```python
from build123d import *

# Parameters (mm, degrees)
SKETCH1_W           = 88
SKETCH1_H           = 51
BOSS_EXTRUDE1_DEPTH = 2
SKETCH2_W           = 60.2
SKETCH2_H           = 45.9
CUT_EXTRUDE1_DEPTH  = 2
SKETCH3_W           = 92
SKETCH3_H           = 55
SKETCH3_W_2         = 88
SKETCH3_H_2         = 51
BOSS_EXTRUDE2_DEPTH = 26


with BuildPart() as part:
    # Sketch1 → Boss-Extrude1 (new body)
    with BuildSketch(Plane(origin=(0, 0, 0), x_dir=(1, 0, 0), z_dir=(0, 1, 0))):
        Rectangle(SKETCH1_W, SKETCH1_H)
    extrude(amount=BOSS_EXTRUDE1_DEPTH)

    # Sketch2 → Cut-Extrude1 (cut)
    with BuildSketch(Plane(origin=(0, 0, 0), x_dir=(1, 0, 0), z_dir=(0, 1, 0))):
        with Locations((-3.6, 0)):
            Rectangle(SKETCH2_W, SKETCH2_H)
    extrude(amount=CUT_EXTRUDE1_DEPTH, mode=Mode.SUBTRACT)

    # Sketch3 → Boss-Extrude2 (add)
    with BuildSketch(Plane(origin=(0, 0, 0), x_dir=(1, 0, 0), z_dir=(0, 1, 0))):
        Rectangle(SKETCH3_W, SKETCH3_H)
        Rectangle(SKETCH3_W_2, SKETCH3_H_2, mode=Mode.SUBTRACT)
    extrude(amount=BOSS_EXTRUDE2_DEPTH)


solid = part.part
```
Geometry: final body of the model. Coordinates: model frame, mm. A direction names the side the tool comes from. Round coordinates to 2 decimals unless told otherwise and drop trailing zeros. Write each loop counter-clockwise with the first axis right and the second up, starting at its lowest first coordinate (ties: lowest second). Pieces come first, ordered by that corner, then holes.
Item 1: Section query D-D (x = -38). Return loops of the section in (y, z), plus the area to 3 significant figures.
Item 2: Pin query (flat end, axial travel): P1, Ø6, axis at x = -17, z = 18, coming from the +Y side. Return the tip coordinate at first contact, or that it passes through.
Item 3: Section query B-B (x = -3). Return loops of the section in (y, z), plus the area to 3 significant figures.
Item 4: Material intervals for L1, parallel to Z at x = -4, y = 4; L2, parallel to X at y = 16.25, z = 20.5; L3, parallel to Y at x = 42, z = 7, sorted ascending.
Item 5: Mould query, pull axis X, two halves, no side actions, for faces 1 (the face through (46, 13, 0)), 2 (the face through (-4, 1, -22.95)), 3 (the face through (-46, 13, 0)), 4 (the face through (-1, 13, -27.5)). Classes: +X half, -X half, draft (parallel to the pull), parting line (faces both ways), or undercut.
Item 6: Section query C-C (z = 10.5). Return loops of the section in (x, y).
Item 7: Section query A-A (y = 23.5). Return loops of the section in (x, z).
Item 8: Set-up query: faces 5 (the face through (-4, 26, 26)), 6 (the face through (-1, 14, 25.5)), 7 (the face through (-33.7, 1, 0)). Return all of +Z, -Z, +X, -X, +Y, -Y with unobstructed straight access to the full face (end or side cutting, diameter ignored); none if empty.
Completed:
1. outline: (0, -27.5) - (26, -27.5) - (26, -25.5) - (2, -25.5) - (2, 25.5) - (26, 25.5) - (26, 27.5) - (0, 27.5) - close
1. area: 206 mm2
2. P1: passes through
3. outline: (0, -27.5) - (26, -27.5) - (26, -25.5) - (2, -25.5) - (2, -22.95) - (0, -22.95) - close; (0, 22.95) - (2, 22.95) - (2, 25.5) - (26, 25.5) - (26, 27.5) - (0, 27.5) - close
3. area: 114 mm2
4. L1: z = -27.5 to -25.5, 25.5 to 27.5
4. L2: x = -46 to -44, 44 to 46
4. L3: y = 0 to 2
5. face 1: +X half
5. face 2: undercut
5. face 3: -X half
5. face 4: draft
6. outline: (-46, 0) - (-33.7, 0) - (-33.7, 2) - (-44, 2) - (-44, 26) - (-46, 26) - close; (26.5, 0) - (46, 0) - (46, 26) - (44, 26) - (44, 2) - (26.5, 2) - close
7. outline: (-46, -27.5) - (46, -27.5) - (46, 27.5) - (-46, 27.5) - close; hole (-44, -25.5) - (44, -25.5) - (44, 25.5) - (-44, 25.5) - close
8. face 5: +Z, -Z, +X, -X, +Y
8. face 6: +Y
8. face 7: +Y, -Y
